Verification items for the finished model (mm, model axes). Face numbers are marked on the shaded views. A direction names the side the tool comes from. Give positions to 0.01 mm unless a question says otherwise; leave off trailing zeros. Order: outer loops, then holes, each group sorted by start corner. A loop starts at its lowest first (then second) coordinate and runs counter-clockwise, first axis right, second up.
(1) Gauge pin test, flat ends, axial feed: pin 1 (4.5 mm diameter, centred on y = 7.5, z = -17, fed in from -X); pin 2 (11 mm diameter, centred on y = 6.56, z = -15, fed in from -X); pin 3 (4 mm diameter, centred on x = 20.5, z = -2.5, fed in from -Y); pin 4 (2 mm diameter, centred on x = 17.5, y = -2.5, fed in from -Z). Record the tip position at first contact, or that the pin passes through.
(2) Scan lines: L1, parallel to Y at x = 27, z = -15 (3 decimals); L2, parallel to Y at x = 26.25, z = -15 (3 decimals); L3, parallel to Z at x = 24.75, y = 15.06 (3 decimals). Record each from-to range of solid material in increasing order.
(3) Sectioned sample at B-B on z = -15. Count the separate pieces of the cut face and the enclosed holes in it, plus the area to 3 significant figures.
(4) Sectioned sample at D-D on y = 54.5. Record the cut outline in (x, z), plus the area to 3 significant figures.
(5) Sectioned sample at A-A on y = 23.56. Record the cut outline in (x, z), plus the area to 3 significant figures.
(6) Access from +Z, -Z, +X, -X, +Y, -Y to the whole of each face (thin tool, end or side, straight path). Record for the marked faces 5, 6, 7 and 8.
(7) Mould release check, pull along Z, two halves, no side actions. Record for the marked faces 1, 2, 3 and 4: pulls with the +Z half, pulls with the -Z half, needs draft (parallel to the pull), parting line crosses it, or undercut.
(8) Sectioned sample at C-C on x = 4. Record the cut outline in (y, z).
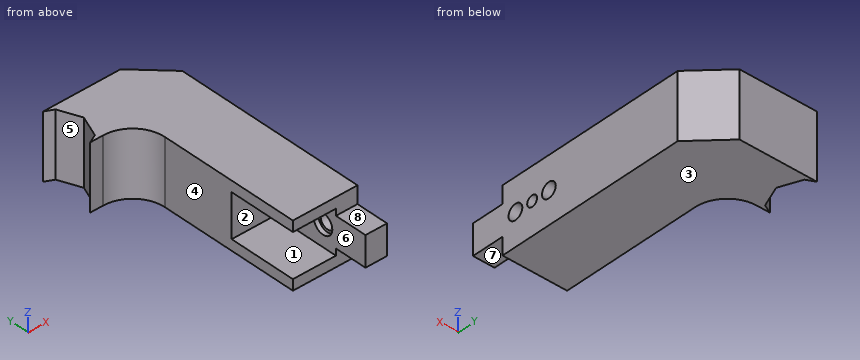
Autodesk Inventor part; units mm, degrees
ref_plane "YZ Plane" through (0, 0, 0) normal (1, 0, 0) x (0, 1, 0)
ref_plane "XZ Plane" through (0, 0, 0) normal (0, 1, 0) x (-1, 0, 0)
ref_plane "XY Plane" through (0, 0, 0) normal (0, 0, 1) x (1, 0, 0)
sketch "Sketch1" plane through (0, 0, 0) normal (0, 0, 1) x (1, 0, 0)
  line L0 (0, 0) -> (25, 0)
  line L1 (25, 0) -> (25, 40)
  line L2 (25, 40) -> (0, 40)
  line L3 (0, 40) -> (0, 0)
  dimension "d1" = 25
  dimension "d2" = 40
  dimension "d3" = 25
extrude "Extrusion1" add sketch "Sketch1" against normal blind 30
sketch "Sketch2" plane through (25, 0, 0) normal (1, 0, 0) x (0, 0, -1)
  line L0 (0, 0) -> (30, 0)
  circle A0 centre (15, 6.56) radius 2.46
extrude "Extrusion2" cut sketch "Sketch2" against normal blind 30
sketch "Sketch3" plane through (0, 0, 0) normal (-1, 0, 0) x (0, 0, 1)
  line L0 (0, 0) -> (-30, 0)
  line L1 (-25.05, 0) -> (-4.95, 0)
  line L2 (-4.95, 0) -> (-4.95, 33.12)
  line L3 (-4.95, 33.12) -> (-25.05, 33.12)
  line L4 (-25.05, 33.12) -> (-25.05, 0)
  dimension "d11" = 20.1
extrude "Extrusion3" cut sketch "Sketch3" against normal blind 20
sketch "Sketch4" plane through (0, 0, 0) normal (0, -1, 0) x (1, 0, 0)
  line L0 (20, -4.95) -> (20, -25.05)
  line L1 (20, -15) -> (25, -15)
  line L2 (25, 0) -> (25, -30)
  line L3 (20, -8.025) -> (25, -8.025)
  line L4 (25, -8.025) -> (25, -21.975)
  line L5 (25, -21.975) -> (20, -21.975)
  line L6 (20, -21.975) -> (20, -8.025)
  line L7 (20, -8.025) -> (25, -21.975) construction
  line L8 (25, -8.025) -> (20, -21.975) construction
  line L9 (25, -12.54) -> (25, -17.46)
  point P0 (0, 0)
  point P1 (22.5, -15)
  dimension "d14" = 13.95
extrude "Extrusion4" add sketch "Sketch4" along normal blind 15
sketch "Sketch5" plane through (20, 0, 0) normal (-1, 0, 0) x (0, 0, 1)
  circle A0 centre (-15, 6.56) radius 2.46
  circle A1 centre (-15, 6.56) radius 4.7025
  circle A2 centre (-15, 6.56) radius 2.46
  circle A3 centre (-15, 6.56) radius 2.46
  point P0 (0, 0)
  dimension "d17" = 9.405
extrude "Extrusion5" cut sketch "Sketch5" against normal blind 2.1
sketch "Sketch6" plane through (25, 0, 0) normal (1, 0, 0) x (0, 0, -1)
  circle A0 centre (15, 6.56) radius 4.7025
  line L0 (15, 6.56) -> (15, 23.56)
  circle A1 centre (15, 23.56) radius 2.46
  point P0 (0, 0)
  dimension "d20" = 17
  dimension "d21" = 4.92
extrude "Extrusion6" cut sketch "Sketch6" against normal blind 10 contours A1
sketch "Sketch7" plane through (20, 0, 0) normal (-1, 0, 0) x (0, 0, 1)
  circle A0 centre (-15, 23.56) radius 2.46
  circle A1 centre (-15, 23.56) radius 4.7025
  point P0 (0, 0)
  dimension "d24" = 9.405
extrude "Extrusion7" cut sketch "Sketch7" against normal blind 2.1
sketch "Sketch9" plane through (25, 0, 0) normal (1, 0, 0) x (0, 0, -1)
  circle A0 centre (15, 6.56) radius 2.46
  circle A1 centre (15, 6.56) radius 2.46
  circle A2 centre (15, 23.56) radius 2.46
  circle A3 centre (15, 23.56) radius 2.46
  line L0 (30, 40) -> (30, 0)
  line L1 (30, 0) -> (30, 40)
  line L2 (30, 40) -> (0, 40)
  line L3 (0, 40) -> (0, 0)
  line L4 (0, 0) -> (8.025, 0)
  line L5 (21.975, 0) -> (21.975, -15)
  line L6 (21.975, -15) -> (8.025, -15)
  line L7 (8.025, -15) -> (8.025, 0)
  line L8 (0, 0) -> (8.025, 0)
  line L9 (21.975, 0) -> (30, 0)
extrude "Extrusion8" add sketch "Sketch9" along normal blind 5
sketch "Sketch10" plane through (0, 40, 0) normal (0, 1, 0) x (1, 0, 0)
  line L0 (0, 30) -> (30, 30)
  line L1 (30, 0) -> (0, 0)
  line L2 (0, 30) -> (30, 30)
  line L3 (30, 30) -> (30, 0)
  line L4 (30, 0) -> (0, 0)
  line L5 (0, 0) -> (0, 30)
extrude "Extrusion9" add sketch "Sketch10" along normal blind 10
sketch "Sketch12" plane through (30, 0, 0) normal (1, 0, 0) x (0, 0, -1)
  circle A0 centre (15, 6.56) radius 2.46
  line L0 (15, 6.56) -> (15, 15.06)
  circle A1 centre (15, 15.06) radius 2.525
  point P0 (0, 0)
  dimension "d31" = 8.5
  dimension "d33" = 5.05
extrude "Extrusion10" cut sketch "Sketch12" against normal blind 30 contours A1
sketch "Sketch14" plane through (0, 0, 0) normal (0, 0, 1) x (1, 0, 0)
  line L0 (30, 50) -> (0, 50)
  line L1 (0, 50) -> (0, 65)
  line L2 (30, 0) -> (30, 50)
  line L3 (30, 89) -> (30, 50)
  arc A0 (0, 65) -> (-15, 80) centre (-15, 65) ccw
  line L4 (30, 85) -> (30, 80)
  line L5 (-21, 104) -> (15, 104)
  line L6 (-17, 102) -> (-21, 104)
  line L7 (-17, 102) -> (-13, 92)
  line L8 (-17, 82) -> (-21, 80)
  line L9 (-17, 82) -> (-13, 92)
  line L10 (30, 89) -> (15, 104)
  line L11 (-15, 80) -> (-21, 80)
  point P0 (0, 0)
  point P1 (0, 80)
  dimension "d47" = 30
  dimension "d54" = 15
  dimension "d77" = 6
extrude "Extrusion12" add sketch "Sketch14" against normal blind 30
sketch "Sketch15" plane through (0, 0, -25.05) normal (-1, 0, 0) x (0, 0, 1)
  line L0 (0, 33.12) -> (20.1, 33.12)
  line L1 (20.1, 33.12) -> (20.1, 0)
  line L2 (0, 33.12) -> (20.1, 33.12)
  line L3 (20.1, 33.12) -> (20.1, 31.1)
  line L4 (20.1, 31.1) -> (0, 31.1)
  line L5 (0, 31.1) -> (0, 33.12)
  point P0 (25.05, 0)
  dimension "d57" = 2.02
extrude "Extrusion13" add sketch "Sketch15" against normal blind 20
sketch "Sketch19" plane through (30, 0, 0) normal (1, 0, 0) x (0, 0, -1)
  circle A0 centre (15, 23.56) radius 2.46
  circle A1 centre (15, 23.56) radius 3.5
  circle A2 centre (15, 6.56) radius 2.46
  circle A3 centre (15, 6.56) radius 3.5
  point P0 (0, 0)
  dimension "d73" = 7
  dimension "d74" = 7
extrude "Extrusion14" cut sketch "Sketch19" against normal blind 10
properties part number "20mm_x_30mm"
Ans:
1. pin 1: stops at x = 22.1
1. pin 2: stops at x = 20
1. pin 3: stops at y = 0
1. pin 4: passes through
2. L1: y = -15 to 3.06, 10.06 to 12.535, 17.585 to 20.06, 27.06 to 92
2. L2: y = -15 to 3.06, 10.06 to 12.535, 17.585 to 20.06, 27.06 to 92.75
2. L3: z = -30 to -17.525, -12.475 to 0
3. separate pieces: 4
3. enclosed holes: 0
3. area: 2,760 mm2
4. outline: (0, -30) - (30, -30) - (30, 0) - (0, 0) - close
4. area: 900 mm2
5. outline: (0, -30) - (30, -30) - (30, -18.5) - (22.1, -18.5) - (22.1, -19.7) - (20, -19.7) - (20, -25.05) - (0, -25.05) - close; (0, -4.95) - (20, -4.95) - (20, -10.3) - (22.1, -10.3) - (22.1, -11.5) - (30, -11.5) - (30, 0) - (0, 0) - close
5. area: 423 mm2
6. face 5: +Z, -Z, -X
6. face 6: -X, -Y
6. face 7: -Z, +X, -X, -Y
6. face 8: +Z, +X, -X, -Y
7. face 1: undercut
7. face 2: undercut
7. face 3: pulls with the -Z half
7. face 4: needs draft
8. outline: (0, -30) - (104, -30) - (104, 0) - (0, 0) - (0, -4.95) - (31.1, -4.95) - (31.1, -25.05) - (0, -25.05) - close
